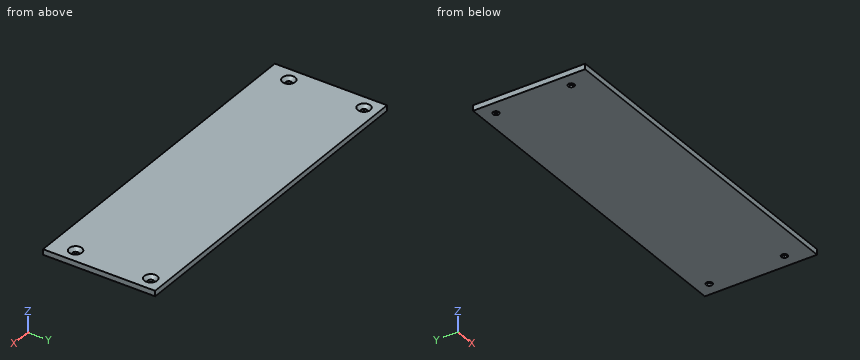
from build123d import *

# Parameters (mm, degrees)
ESQUISSE1_W                                 = 249
ESQUISSE1_H                                 = 82
BOSS_EXTRU_1_DEPTH                          = 4
FRAISAGE_POUR_VIS_T_TE_FRAIS_E_M42_AT_COUNT = 2
FRAISAGE_POUR_VIS_T_TE_FRAIS_E_M42_AT_PITCH = 55
FRAISAGE_POUR_VIS_T_TE_FRAIS_E_M42_2_COUNT  = 2
FRAISAGE_POUR_VIS_T_TE_FRAIS_E_M42_2_PITCH  = 229
FRAISAGE_POUR_VIS_T_TE_FRAIS_E_M42_3_COUNT  = 2
FRAISAGE_POUR_VIS_T_TE_FRAIS_E_M42_3_PITCH  = 235.512207752


with BuildPart() as part:
    # Esquisse1 → Boss.-Extru.1 (new body)
    with BuildSketch(Plane.XY):
        Rectangle(ESQUISSE1_W, ESQUISSE1_H)
    extrude(amount=BOSS_EXTRU_1_DEPTH)

    # Esquisse6 → Fraisage pour vis à tête fraisée M42 (revolve, cut)
    with BuildSketch(Plane(origin=(-114.5, -24, 4), x_dir=(0, -1, 0), z_dir=(1, 0, 0))):
        Polygon((0, 0), (0, 4), (2.25, 4), (2.25, 2.45), (4.7, 0), align=None)
    fraisage_pour_vis_t_te_frais_e_m42 = revolve(axis=Axis((-114.5, -24, 10.35), (0, 0, -1)), mode=Mode.SUBTRACT)

    # Fraisage pour vis à tête fraisée M42 at: Fraisage pour vis à tête fraisée M42 ×2
    with Locations(*[(0, i * FRAISAGE_POUR_VIS_T_TE_FRAIS_E_M42_AT_PITCH, 0) for i in range(1, FRAISAGE_POUR_VIS_T_TE_FRAIS_E_M42_AT_COUNT)]):
        add(fraisage_pour_vis_t_te_frais_e_m42, mode=Mode.SUBTRACT)

    # Fraisage pour vis _ t_te frais_e M42 2: Fraisage pour vis à tête fraisée M42 ×2
    with Locations(*[(i * FRAISAGE_POUR_VIS_T_TE_FRAIS_E_M42_2_PITCH, 0, 0) for i in range(1, FRAISAGE_POUR_VIS_T_TE_FRAIS_E_M42_2_COUNT)]):
        add(fraisage_pour_vis_t_te_frais_e_m42, mode=Mode.SUBTRACT)

    # Fraisage pour vis _ t_te frais_e M42 3: Fraisage pour vis à tête fraisée M42 ×2
    with Locations(*[Vector(0.972348747, 0.233533542, 0) * (i * FRAISAGE_POUR_VIS_T_TE_FRAIS_E_M42_3_PITCH) for i in range(1, FRAISAGE_POUR_VIS_T_TE_FRAIS_E_M42_3_COUNT)]):
        add(fraisage_pour_vis_t_te_frais_e_m42, mode=Mode.SUBTRACT)


solid = part.part
Model file for the job. Use its own axes, mm. Round coordinates to 2 decimals unless told otherwise and drop trailing zeros. Loops run counter-clockwise (first coordinate to the right, second up) from the corner with the lowest first, then second, coordinate; pieces in that order, holes last. Notation, with made-up numbers: (18, 36) - (57, 36) arc R15 ccw to (57, 45) - close; hole circle Ø3 at (-8.5, 61). An arc over 180 degrees is marked (long way). Write each question's results on one line, items separated by ' | '.
(1) Pin check, flat tips, straight feed: pin 1 (5 mm diameter, centred on x = -114.5, y = 31, fed in from +Z); pin 2 (4 mm diameter, centred on x = -114.5, y = -24, fed in from +Z). Stop position of each tip, or through.
Answer below:
pin 1: stops at z = 1.8 | pin 2: passes through
(2) Wall check: L1, parallel to X at y = -24, z = 0.9; L2, parallel to Y at x = -114.5, z = 1; L3, parallel to X at y = 30, z = 3.05. Give the ranges that are in metal, low to high.
Answer below:
L1: x = -124.5 to -116.75, -112.25 to 112.25, 116.75 to 124.5 | L2: y = -41 to -26.25, -21.75 to 28.75, 33.25 to 41 | L3: x = -124.5 to -118.11, -110.89 to 110.89, 118.11 to 124.5
(3) Saw through at B-B, the plane x = 114.5. List the corners of the cut face in (y, z), then the cut area to 3 significant figures.
Answer below:
outline: (-41, 0) - (-26.25, 0) - (-26.25, 1.55) - (-28.7, 4) - (-41, 4) - close; (-21.75, 0) - (28.75, 0) - (28.75, 1.55) - (26.3, 4) - (-19.3, 4) - (-21.75, 1.55) - close; (33.25, 0) - (41, 0) - (41, 4) - (35.7, 4) - (33.25, 1.55) - close | area: 280 mm^2
(4) Saw through at A-A, the plane y = -24. List the corners of the cut face in (x, z).
Answer below:
outline: (-124.5, 0) - (-116.75, 0) - (-116.75, 1.55) - (-119.2, 4) - (-124.5, 4) - close; (-112.25, 0) - (112.25, 0) - (112.25, 1.55) - (109.8, 4) - (-109.8, 4) - (-112.25, 1.55) - close; (116.75, 0) - (124.5, 0) - (124.5, 4) - (119.2, 4) - (116.75, 1.55) - close
